Input: part model. Units: mm. Frame: model coordinates. Face numbers are marked on the shaded views. A direction names the side the tool comes from. Round coordinates to 2 decimals unless told otherwise and drop trailing zeros. Order: outer loops, then holes, each group sorted by start corner. A loop starts at its lowest first (then second) coordinate and runs counter-clockwise, first axis right, second up. Notation, with made-up numbers: (-35.75, -26.75) -> (-16.75, -26.75) arc R16 ccw to (-16.75, 1.25) -> close; hole circle Ø3 at (36.25, 74). An arc over 180 degrees is marked (long way). Answer as CSV lines item,"result". Start each with the question number.
1) Section query D-D, the plane z = 10. Output: boundary loops of the cut face in (x, y), and give its area (3 significant figures).
2) Section query C-C, the plane z = 39.5. Output: boundary loops of the cut face in (x, y), and give its area (3 significant figures).
3) First-contact query: P1, Ø4, axis at x = -40.5, y = 124, coming from the +Z side; P2, Ø2, axis at x = 23.5, y = 299, coming from the -Z side; P3, Ø9.5, axis at x = 60.5, z = 57, coming from the +Y side; P4, Ø1, axis at x = -49.5, z = 68.5, coming from the -Y side. Flat tips, straight axial feed; report the tip coordinate or a pass-through.
4) Section query B-B, the plane x = 16. Output: boundary loops of the cut face in (y, z), and give its area (3 significant figures).
5) Mould query, pull axis X, two halves, no side actions, for the marked faces 4, 5 and 6. Classes: +X half, -X half, draft (parallel to the pull), parting line (faces both ways), or undercut.
6) Section query A-A, the plane y = 146.5. Output: boundary loops of the cut face in (x, z), and give its area (3 significant figures).
7) Line query: L1, parallel to Z at x = 52.5, y = 27; L2, parallel to X at y = 359.5, z = 29.5; L3, parallel to X at y = 216, z = 38.5. Output: solid intervals per line, ascending.
8) Access query for the marked faces 1, 2 and 3. Directions: +Z, -Z, +X, -X, +Y, -Y. A direction counts if a zero-diameter tool reaches every point of the face in a straight line with its end or side. Return the directions, or none.
```python
from build123d import *

# Parameters (mm, degrees)
BOSS_EXTRUDE1_DEPTH = 390
CUT_EXTRUDE2_DEPTH  = 14
CUT_EXTRUDE3_DEPTH  = 50
BOSS_EXTRUDE2_DEPTH = 10
BOSS_EXTRUDE4_START = 22
BOSS_EXTRUDE4_DEPTH = 78
SKETCH22_R          = 2.1
CUT_EXTRUDE4_DEPTH  = 15
SKETCH23_R          = 3.1
CUT_EXTRUDE5_DEPTH  = 60


with BuildPart() as part:
    # Sketch1 → Boss-Extrude1 (new body)
    with BuildSketch(Plane(origin=(0, 0, 0), x_dir=(1, 0, 0), z_dir=(0, 1, 0))):
        with BuildLine():
            Line((-10, -5.773502692), (-86.602540378, -50))
            Line((-86.602540378, -50), (-79.102540378, -62.990381057))
            Line((-79.102540378, -62.990381057), (-53.121778265, -47.990381057))
            Line((-53.121778265, -47.990381057), (-50.621778265, -52.320508076))
            Line((-50.621778265, -52.320508076), (-76.602540378, -67.320508076))
            Line((-76.602540378, -67.320508076), (-66.602540378, -84.641016151))
            Line((-66.602540378, -84.641016151), (0, -46.188021535))
            Line((0, -46.188021535), (66.602540378, -84.641016151))
            Line((66.602540378, -84.641016151), (76.602540378, -67.320508076))
            Line((76.602540378, -67.320508076), (50.621778265, -52.320508076))
            Line((50.621778265, -52.320508076), (53.121778265, -47.990381057))
            Line((53.121778265, -47.990381057), (79.102540378, -62.990381057))
            Line((79.102540378, -62.990381057), (86.602540378, -50))
            Line((86.602540378, -50), (10, -5.773502692))
            ThreePointArc((10, -5.773502692), (0, -3.094010768), (-10, -5.773502692))
        make_face()
    extrude(amount=BOSS_EXTRUDE1_DEPTH)

    # Sketch18 → Cut-Extrude2 (cut)
    with BuildSketch(Plane.XZ):
        Polygon((-76.602540378, 67.320508076), (0, 23.094010768), (76.602540378, 67.320508076), (66.602540378, 84.641016151), (0, 46.188021535), (-66.602540378, 84.641016151), align=None)
    extrude(amount=-CUT_EXTRUDE2_DEPTH, mode=Mode.SUBTRACT)

    # Sketch19 → Cut-Extrude3 (cut)
    with BuildSketch(Plane(origin=(0, 390, 0), x_dir=(1, 0, 0), z_dir=(0, 1, 0))):
        Polygon((76.602540378, -67.320508076), (0, -23.094010768), (-76.602540378, -67.320508076), (-79.102540378, -62.990381057), (0, -17.320508076), (79.102540378, -62.990381057), align=None)
    extrude(amount=-CUT_EXTRUDE3_DEPTH, mode=Mode.SUBTRACT)

    # Sketch20 → Boss-Extrude2 (add)
    with BuildSketch(Plane.XZ):
        Polygon((76.602540378, 67.320508076), (50.621778265, 52.320508076), (53.121778265, 47.990381057), (79.102540378, 62.990381057), align=None)
        Polygon((-50.621778265, 52.320508076), (-76.602540378, 67.320508076), (-79.102540378, 62.990381057), (-53.121778265, 47.990381057), align=None)
    extrude(amount=-BOSS_EXTRUDE2_DEPTH)

    # Boss-Extrude3: read off the stored shape, not the designer's step
    # Boss-Extrude3: loft between two sections, ruled curve by curve
    boss_extrude3_from = [
        Edge.make_line((-53.612159322, 357.320508076, 107.141016151), (0, 357.320508076, 76.188021535)),
        Edge.make_line((-53.612159322, 368.206188758, 107.141016151), (0, 368.206188758, 76.188021535)),
        Edge.make_line((0, 368.206188758, 76.188021535), (0, 357.320508076, 76.188021535)),
        Edge.make_line((-53.612159322, 368.206188758, 107.141016151), (-53.612159322, 357.320508076, 107.141016151)),
    ]
    boss_extrude3_to = [
        Edge.make_line((-66.602540378, 340, 84.641016151), (0, 340, 46.188021535)),
        Edge.make_line((-66.602540378, 375, 84.641016151), (0, 375, 46.188021535)),
        Edge.make_line((0, 375, 46.188021535), (0, 340, 46.188021535)),
        Edge.make_line((-66.602540378, 375, 84.641016151), (-66.602540378, 340, 84.641016151)),
    ]
    boss_extrude3 = Solid(Shell([*[Face.make_surface_from_curves(boss_extrude3_from[k], boss_extrude3_to[k]) for k in range(4)], Face(Wire(boss_extrude3_from)), Face(Wire(boss_extrude3_to))]))
    add(boss_extrude3)

    # Boss-Extrude4: read off the stored shape, not the designer's step
    # Boss-Extrude4 outline → Boss-Extrude4 (add)
    with BuildSketch(Plane(origin=(0, 0, 0), x_dir=(0.49999999999999767, 0, -0.86602540378444), z_dir=(0.8660254037844399, 0, 0.49999999999999795)).offset(BOSS_EXTRUDE4_START)):
        Polygon((-65.980762114, 357.320508076), (-40, 340), (-40, 375), (-65.980762114, 368.206188758), align=None)
    extrude(amount=BOSS_EXTRUDE4_DEPTH)

    # Sketch22 → Cut-Extrude4 (cut)
    with BuildSketch(Plane(origin=(47.172106066, 360.789319124, 81.704484407), x_dir=(0.9919674102096397, -0.12336978823439819, -0.027938368473838716), z_dir=(0.12649370372465277, 0.9674695714450555, 0.21909352168866233))):
        with Locations(Location((-89.639756751, -1.109544744, 0), (0, 0, 270))):
            Circle(SKETCH22_R)
    cut_extrude4 = extrude(amount=-CUT_EXTRUDE4_DEPTH, mode=Mode.SUBTRACT)

    # Mirror1: Cut-Extrude4 across plane
    add(cut_extrude4.mirror(Plane(origin=(0, 0, 0), x_dir=(0, 0, 1), z_dir=(1, 0, 0))), mode=Mode.SUBTRACT)

    # Sketch23 → Cut-Extrude5 (cut)
    with BuildSketch(Plane.XZ.offset(-14)):
        with Locations(Location((-25.980762114, 49.641016151, 0), (0, 0, 270))):
            Circle(SKETCH23_R)
        with Locations(Location((-51.961524227, 64.641016151, 0), (0, 0, 270))):
            Circle(SKETCH23_R)
    cut_extrude5 = extrude(amount=-CUT_EXTRUDE5_DEPTH, mode=Mode.SUBTRACT)

    # Mirror2: Cut-Extrude5 across plane
    add(cut_extrude5.mirror(Plane(origin=(0, 0, 0), x_dir=(0, 0, 1), z_dir=(1, 0, 0))), mode=Mode.SUBTRACT)


solid = part.part
```
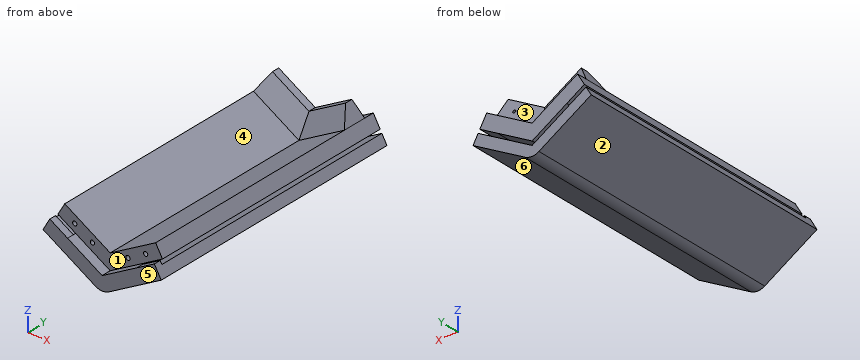
Findings:
1,outline,"(-17.32, 0) -> (17.32, 0) -> (17.32, 390) -> (-17.32, 390) -> close"
1,area,"13,500 mm^2"
2,outline,"(-68.42, 0) -> (-28.42, 0) -> (-28.42, 14) -> (28.42, 14) -> (28.42, 0) -> (68.42, 0) -> (68.42, 390) -> (38.42, 390) -> (38.42, 340) -> (28.42, 340) -> (28.42, 390) -> (-28.42, 390) -> (-28.42, 340) -> (-38.42, 340) -> (-38.42, 390) -> (-68.42, 390) -> close"
2,area,"51,600 mm^2"
3,P1,"stops at z = 70.73"
3,P2,"stops at z = 12.99"
3,P3,"stops at y = 390"
3,P4,"stops at y = 14"
4,outline,"(0, 9.24) -> (390, 9.24) -> (390, 26.56) -> (340, 26.56) -> (340, 32.33) -> (390, 32.33) -> (390, 55.43) -> (375, 55.43) -> (368.21, 85.43) -> (357.32, 85.43) -> (340, 55.43) -> (14, 55.43) -> (14, 32.33) -> (0, 32.33) -> close"
4,area,"18,100 mm^2"
5,face 4,"undercut"
5,face 5,"draft"
5,face 6,"+X half"
6,outline,"(-86.6, 50) -> (-10, 5.77) arc R20 ccw to (10, 5.77) -> (86.6, 50) -> (79.1, 62.99) -> (53.12, 47.99) -> (50.62, 52.32) -> (76.6, 67.32) -> (66.6, 84.64) -> (0, 46.19) -> (-66.6, 84.64) -> (-76.6, 67.32) -> (-50.62, 52.32) -> (-53.12, 47.99) -> (-79.1, 62.99) -> close"
6,area,"6,750 mm^2"
7,L1,"z = 30.31 to 49.07, 53.4 to 61.59, 67.69 to 76.5"
7,L2,"x = -51.1 to -21.1, -11.1 to 11.1, 21.1 to 51.1"
7,L3,"x = -66.68 to 66.68"
8,face 1,"+Z, -Y"
8,face 2,"-Z, -X, +Y, -Y"
8,face 3,"+Z, +Y"
